Verification items for this drawing (mm, ordinates from the low corner). A direction names the side the tool comes from. Coordinates: 2 decimals unless noted, no trailing zeros. Write each loop counter-clockwise with the first axis right and the second up, starting at its lowest first coordinate (ties: lowest second). Pieces come first, ordered by that corner, then holes.
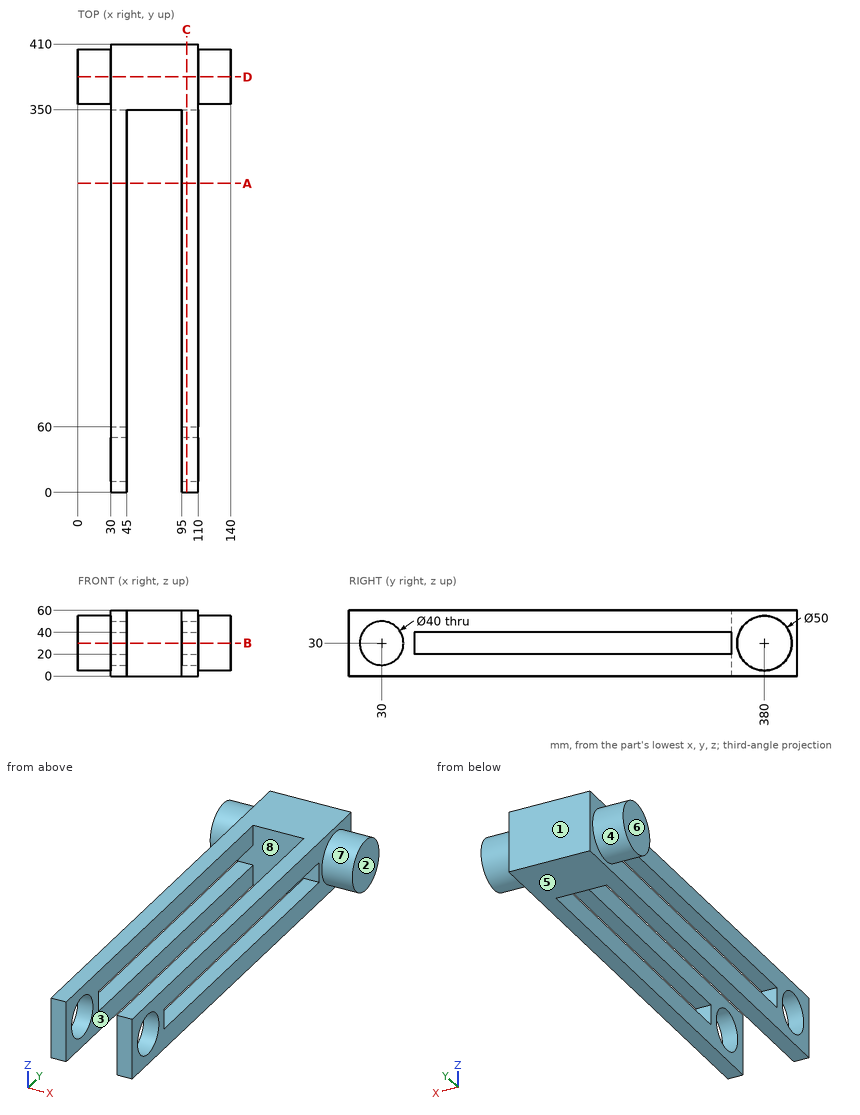
1. Sectioned sample at D-D, the plane y = 380. Record the boundary of the cut face in (x, z).
Computed values:
outline: (0, 5) - (30, 5) - (30, 0) - (110, 0) - (110, 5) - (140, 5) - (140, 55) - (110, 55) - (110, 60) - (30, 60) - (30, 55) - (0, 55) - close
2. Gauge pin test, flat ends, axial feed: pin 1 Ø5 at (x, y) = (107.5, 102) entering from -Z; pin 2 Ø2 at (y, z) = (217, 17) entering from +X; pin 3 Ø8 at (x, z) = (80.5, 38.5) entering from -Y; pin 4 Ø24 at (y, z) = (30, 30) entering from +X. Record the tip position at first contact, or that the pin passes through.
Computed values:
pin 1: stops at z = 0
pin 2: stops at x = 110
pin 3: stops at y = 350
pin 4: passes through
3. Access from +Z, -Z, +X, -X, +Y, -Y to the whole of each face (thin tool, end or side, straight path). Record for the marked faces 4, 5, 6, 7 and 8.
Computed values:
face 4: -X
face 5: -Z, +X, -X, +Y, -Y
face 6: +Z, -Z, -X, +Y, -Y
face 7: +X
face 8: none
4. Sectioned sample at A-A, the plane y = 282.5. Record the boundary of the cut face in (x, z), and give its area (3 significant figures).
Computed values:
outline: (30, 0) - (45, 0) - (45, 20) - (30, 20) - close; (30, 40) - (45, 40) - (45, 60) - (30, 60) - close; (95, 0) - (110, 0) - (110, 20) - (95, 20) - close; (95, 40) - (110, 40) - (110, 60) - (95, 60) - close
area: 1,200 mm2
5. Sectioned sample at B-B, the plane z = 30. Record the boundary of the cut face in (x, y), and give its area (3 significant figures).
Computed values:
outline: (0, 355) - (30, 355) - (30, 350) - (110, 350) - (110, 355) - (140, 355) - (140, 405) - (110, 405) - (110, 410) - (30, 410) - (30, 405) - (0, 405) - close; (30, 0) - (45, 0) - (45, 10) - (30, 10) - close; (30, 50) - (45, 50) - (45, 60) - (30, 60) - close; (95, 0) - (110, 0) - (110, 10) - (95, 10) - close; (95, 50) - (110, 50) - (110, 60) - (95, 60) - close
area: 8,400 mm2
6. Draft check along X on the marked faces 1, 2 and 3. Enter one of: released by +X, released by -X, zero draft, split by the parting line, or undercut.
Computed values:
face 1: zero draft
face 2: released by +X
face 3: undercut
7. Thickness scan on line 1 along X through (y, z) = (292.5, 11); line 2 along Y through (x, z) = (36, 24.5); line 3 along Z through (x, y) = (106, 30). Record the ranges inside material, lowest first.
Computed values:
line 1: x = 30 to 45, 95 to 110
line 2: y = 0 to 10.77, 49.23 to 60, 350 to 410
line 3: z = 0 to 10, 50 to 60
8. Sectioned sample at C-C, the plane x = 99.5. Record the boundary of the cut face in (y, z).
Computed values:
outline: (0, 0) - (410, 0) - (410, 60) - (0, 60) - close; hole circle Ø40 at (30, 30); hole (60, 20) - (350, 20) - (350, 40) - (60, 40) - close
